Geometry check sheet. Reference: the model listing, model coordinates, mm. A direction names the side the tool comes from. Coordinates: 2 decimals unless noted, no trailing zeros. Write each loop counter-clockwise with the first axis right and the second up, starting at its lowest first coordinate (ties: lowest second). Pieces come first, ordered by that corner, then holes. Notation, with made-up numbers: (85, -18) -> (138, -18) arc R17 cw to (138, -3) -> close; hole circle Ø4 at (-26, 9). An arc over 180 degrees is marked (long way). One line per question, with ' | ' between items.
Autodesk Inventor part; units mm, degrees
ref_plane "YZ Plane" through (0, 0, 0) normal (1, 0, 0) x (0, 1, 0)
ref_plane "XZ Plane" through (0, 0, 0) normal (0, 1, 0) x (-1, 0, 0)
ref_plane "XY Plane" through (0, 0, 0) normal (0, 0, 1) x (1, 0, 0)
sketch "Эскиз1" plane through (0, 0, 0) normal (0, 0, 1) x (1, 0, 0)
  line L0 (0, 0) -> (0, 15)
  line L1 (0, 12.5) -> (3, 12.5)
  line L2 (2.1504, 2) -> (4.0415, 2)
  line L3 (2.5, 5) -> (4.0415, 5)
  line L4 (2.5, 6.5) -> (3, 6.5)
  line L5 (0, 0) -> (0.75, 0)
  line L6 (2.5, 6.5) -> (2.5, 5)
  line L7 (3, 12.5) -> (3, 6.5)
  line L8 (0.75, 0) -> (2.1504, 2)
  line L9 (4.0415, 5) -> (4.0415, 2)
  line L10 (0, 12.5) -> (0, 0)
  dimension "d0" = 15
  dimension "d1" = 12.5
  dimension "d2" = 10.5
  dimension "d3" = 7.5
  dimension "d4" = 6
  dimension "d6" = 5
  dimension "d7" = 6
  dimension "d8" = 125
  dimension "d11" = 8.083
  dimension "d44" = 1.5
revolve "Вращение1" add sketch "Эскиз1" angle 360 about axis through (0, 0, 0) along (0, 1, 0)
chamfer "Фаска1" distance 0.25 angle 45 2 edges at (-3, 12.5, 0) (-3, 6.5, 0)
thread "Резьба1"
sketch "Эскиз2" plane through (0, 12.5, 0) normal (0, 1, 0) x (1, 0, 0)
  point P0 (0, 0)
  point P1 (0, 0)
sketch "Эскиз3" plane through (0, 0, 0) normal (0, -1, 0) x (1, 0, 0)
  point P0 (0, 0)
  point P1 (0, 0)
hole "Отверстие2" at (0, 12.5, 0) direction (0, -1, 0) diameter 2 depth 11.3 tip angle 130
chamfer "Фаска2" distance 0.2 angle 45 1 edges at (0, 12.5, -1)
hole "Отверстие3" at (0, 0, 0) direction (0, 1, 0) diameter 0.6 depth 1.2
sketch "Эскиз4" plane through (0, 2, 0) normal (0, -1, 0) x (1, 0, 0)
  circle A0 centre (0, 0) radius 0.3
  circle A1 centre (0, 0) radius 4.0415
  line L0 (4.0415, 0) -> (2.0208, -3.5)
  line L1 (2.0208, -3.5) -> (-2.0207, -3.5)
  line L2 (-2.0207, -3.5) -> (-4.0415, 0)
  line L3 (-4.0415, 0) -> (-2.0208, 3.5)
  line L4 (-2.0208, 3.5) -> (2.0207, 3.5)
  line L5 (2.0207, 3.5) -> (4.0415, 0)
extrude "Выдавливание1" cut sketch "Эскиз4" against normal blind 3 contours L5 A1 | A1 L0 | L4 A1 | A1 L1 | L3 A1 | A1 L2
properties part number "nozzle-0,5"
(1) Cross-section at C-C (y = 5.75). Record the cut outline in (x, z), plus the area to 3 significant figures.
Answers below:
outline: circle Ø5 at (0, 0); hole circle Ø2 at (0, 0) | area: 16.5 mm²
(2) Depth check by flat-ended pin: P1, Ø3, axis at x = -1, z = 1, coming from the -Y side. Enter the tip coordinate at first touch or a pass-through.
Answers below:
P1: stops at y = 0
(3) Material ranges on line 1 (X direction, y = 5.75, z = 0); line 2 (X direction, y = 7.5, z = 0), recorded low to high.
Answers below:
line 1: x = -2.5 to -1, 1 to 2.5 | line 2: x = -3 to -1, 1 to 3
(4) Cross-section at D-D (x = 3.5). Record the cut outline in (y, z).
Answers below:
outline: (2, -0.94) -> (5, -0.94) -> (5, 0.94) -> (2, 0.94) -> close
(5) Tool access check on faces 1 (the face through (0.95, 0.35, -0.3)), 2 (the face through (3, 5, 0)), 3 (the face through (-3, 9, 0)). Record the directions out of +Z, -Z, +X, -X, +Y, -Y that give a thin tool (end or side, any length) a straight path to the whole face; none if there is none.
Answers below:
face 1: -Y | face 2: none | face 3: +Y
(6) Cross-section at B-B (y = 2.5). Record the cut outline in (x, z).
Answers below:
outline: (-4.04, 0) -> (-2.02, -3.5) -> (2.02, -3.5) -> (4.04, 0) -> (2.02, 3.5) -> (-2.02, 3.5) -> close; hole circle Ø2 at (0, 0)
(7) Draft check along Z on faces 4 (the face through (1, 7, 0)), 5 (the face through (-3, 3.5, -1.8)), 6 (the face through (-3.045, 3.479, 1.725)). Enter one of: pulls with the +Z half, pulls with the -Z half, needs draft (parallel to the pull), parting line crosses it, or undercut.
Answers below:
face 4: undercut | face 5: pulls with the -Z half | face 6: pulls with the +Z half
